Check sheet for the modelled part. Datum: model origin and axes. Units: mm. Give positions to 0.01 mm unless a question says otherwise; leave off trailing zeros. Loops run counter-clockwise (first coordinate to the right, second up) from the corner with the lowest first, then second, coordinate; pieces in that order, holes last. Notation, with made-up numbers: (87, 53) - (132, 53) arc R19 cw to (132, 79) - close; hole circle Ø9 at (8, 60.25). An arc over 180 degrees is marked (long way). Answer in a Markdown table with one row per item. Add a question column.
(1) Sectioned sample at B-B on z = 3.4. Enter the section's corners in (x, y).
(2) Sectioned sample at C-C on x = 72. Enter the section's corners in (y, z).
(3) Thickness scan on L1, parallel to X at y = 10, z = 0.55; L2, parallel to Y at x = -111.5, z = 0.8. Record the ranges inside material, lowest first.
(4) Sectioned sample at A-A on y = 40.5. Enter the section's corners in (x, z), then the cut area to 3 significant figures.
from build123d import *

# Parameters (mm, degrees)
SKETCH_W    = 302
SKETCH_H    = 112
SKETCH_W_2  = 287
SKETCH_H_2  = 97
PAD_DEPTH   = 4
FILLET_R    = 1
FILLET001_R = 1
FILLET002_R = 1
FILLET003_R = 1
FILLET004_R = 1
FILLET005_R = 1
FILLET006_R = 1
FILLET007_R = 1


with BuildPart() as part:
    # Sketch → Pad (new body)
    with BuildSketch(Plane.XY):
        Rectangle(SKETCH_W, SKETCH_H)
        Rectangle(SKETCH_W_2, SKETCH_H_2, mode=Mode.SUBTRACT)
    extrude(amount=PAD_DEPTH)

    # Fillet
    fillet_edges = [part.edges().sort_by_distance(p)[0] for p in [
        (-151, -56, 2),
    ]]
    fillet(fillet_edges, radius=FILLET_R)

    # Fillet001
    fillet001_edges = [part.edges().sort_by_distance(p)[0] for p in [
        (151, -56, 2),
    ]]
    fillet(fillet001_edges, radius=FILLET001_R)

    # Fillet002
    fillet002_edges = [part.edges().sort_by_distance(p)[0] for p in [
        (-143.5, 48.5, 2),
    ]]
    fillet(fillet002_edges, radius=FILLET002_R)

    # Fillet003
    fillet003_edges = [part.edges().sort_by_distance(p)[0] for p in [
        (151, 56, 2),
    ]]
    fillet(fillet003_edges, radius=FILLET003_R)

    # Fillet004
    fillet004_edges = [part.edges().sort_by_distance(p)[0] for p in [
        (-151, 56, 2),
    ]]
    fillet(fillet004_edges, radius=FILLET004_R)

    # Fillet005
    fillet005_edges = [part.edges().sort_by_distance(p)[0] for p in [
        (143.5, -48.5, 2),
    ]]
    fillet(fillet005_edges, radius=FILLET005_R)

    # Fillet006
    fillet006_edges = [part.edges().sort_by_distance(p)[0] for p in [
        (143.5, 48.5, 2),
    ]]
    fillet(fillet006_edges, radius=FILLET006_R)

    # Fillet007
    fillet007_edges = [part.edges().sort_by_distance(p)[0] for p in [
        (-143.5, -48.5, 2),
    ]]
    fillet(fillet007_edges, radius=FILLET007_R)


solid = part.part
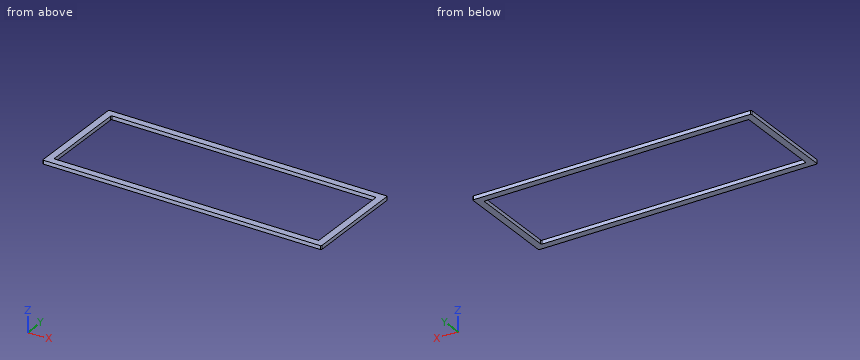
Reply:
| question | item | result |
|---|---|---|
| 1 | outline | (-151, -55) arc R1 ccw to (-150, -56) - (150, -56) arc R1 ccw to (151, -55) - (151, 55) arc R1 ccw to (150, 56) - (-150, 56) arc R1 ccw to (-151, 55) - close; hole (-143.5, -47.5) arc R1 ccw to (-142.5, -48.5) - (142.5, -48.5) arc R1 ccw to (143.5, -47.5) - (143.5, 47.5) arc R1 ccw to (142.5, 48.5) - (-142.5, 48.5) arc R1 ccw to (-143.5, 47.5) - close |
| 2 | outline | (-56, 0) - (-48.5, 0) - (-48.5, 4) - (-56, 4) - close; (48.5, 0) - (56, 0) - (56, 4) - (48.5, 4) - close |
| 3 | L1 | -151 to -143.5, 143.5 to 151 |
| 3 | L2 | -56 to -48.5, 48.5 to 56 |
| 4 | outline | (-151, 0) - (-143.5, 0) - (-143.5, 4) - (-151, 4) - close; (143.5, 0) - (151, 0) - (151, 4) - (143.5, 4) - close |
| 4 | area | 60.0 mm^2 |
